Design review of the part built by this model. Coordinates are the model's own, in mm. A direction names the side the tool comes from. Give positions to 0.01 mm unless a question says otherwise; leave off trailing zeros. Write each loop counter-clockwise with the first axis right and the second up, starting at its lowest first coordinate (ties: lowest second). Pieces come first, ordered by that corner, then holes. Notation, with made-up numbers: M 83.5,-8 L 123.5,-8 A27 ccw 123.5,20 Z; hole C 24,58.25 d4. An arc over 180 degrees is marked long. Use one line per item in the form item = value. Start each with the question number.
from build123d import *

# Parameters (mm, degrees)
SKETCH2_W               = 30
SKETCH2_H               = 30
BOSS_EXTRUDE1_DEPTH     = 36
BOSS_EXTRUDE2_DEPTH     = 80
SKETCH5_R               = 4.1
CUT_EXTRUDE1_DEPTH      = 80
CUT_EXTRUDE2_DEPTH      = 80
CUT_EXTRUDE2_DEPTH_BACK = 80
CHAMFER1_SIZE           = 5


with BuildPart() as part:
    # Sketch2 → Boss-Extrude1 (new body)
    with BuildSketch(Plane(origin=(0, 0, 0), x_dir=(1, 0, 0), z_dir=(0, 1, 0))):
        Rectangle(SKETCH2_W, SKETCH2_H)
    extrude(amount=BOSS_EXTRUDE1_DEPTH)

    # Sketch4 → Boss-Extrude2 (add)
    with BuildSketch(Plane(origin=(15, 0, 0), x_dir=(0, 0, -1), z_dir=(1, 0, 0))):
        Polygon((-8.392439038, 4), (-3, 0), (0, 0), (3, 0), (7.607560962, 4), align=None)
    extrude(amount=BOSS_EXTRUDE2_DEPTH)

    # Sketch5 → Cut-Extrude1 (cut)
    with BuildSketch(Plane(origin=(15, 0, 0), x_dir=(0, 0, -1), z_dir=(1, 0, 0))):
        with Locations((0, 9)):
            Circle(SKETCH5_R)
    extrude(amount=-CUT_EXTRUDE1_DEPTH, mode=Mode.SUBTRACT)

    # Sketch6 → Cut-Extrude2 (cut, two sides)
    with BuildSketch(Plane(origin=(15, 0, 0), x_dir=(0, 0, -1), z_dir=(1, 0, 0))) as cut_extrude2_sk:
        with BuildLine():
            Line((2.528554435, 36.330541101), (-2.528554435, 36.330541101))
            Line((-2.528554435, 36.330541101), (-2.528554435, 29.330704688))
            ThreePointArc((-2.528554435, 29.330704688), (-5.755916854, 22.704075168), (0, 18.1))
            ThreePointArc((0, 18.1), (5.755916854, 22.704075168), (2.528554435, 29.330704688))
            Line((2.528554435, 29.330704688), (2.528554435, 36.330541101))
        make_face()
    extrude(amount=CUT_EXTRUDE2_DEPTH, mode=Mode.SUBTRACT)
    extrude(cut_extrude2_sk.sketch, amount=-CUT_EXTRUDE2_DEPTH_BACK, mode=Mode.SUBTRACT)

    # Chamfer1
    chamfer1_edges = [part.edges().sort_by_distance(p)[0] for p in [
        (0, 36, 15),
        (15, 36, -8.764277217),
        (15, 36, 8.764277217),
        (15, 18, 15),
        (15, 18, -15),
        (0, 36, -15),
    ]]
    chamfer(chamfer1_edges, length=CHAMFER1_SIZE)


solid = part.part
1. We need section A-A (y = 9). State the section outline as (x, z) points, and give its area (3 significant figures).
2. For faces 4 (the flat face through (0, 33, 2.529)), 5 (the flat face through (-3, 36, -6)), 6 (the flat face through (54, 4, 0)), list the 3-axis set-ups (+Z, -Z, +X, -X, +Y, -Y) from which the entire face can be reached by the end or side of a thin tool; tool diameter is ignored.
3. Clearance check with flat-ended pins moving along their axes: pin 1 Ø6 at (y, z) = (9, 4) entering from +X; pin 2 Ø10 at (x, z) = (81, 6) entering from +Y; pin 3 Ø12 at (x, z) = (27.5, -0.5) entering from -Y; pin 4 Ø4 at (x, z) = (73.5, -10.5) entering from +Y. State where each tip first meets the part, or that it passes through.
4. Draft analysis for pull direction Z (two halves, no side actions). For faces 1 (the flat face through (54.44, 1.97, -5.27)), 2 (the cylindrical face through (0.2, 5, 0.9)), 3 (the flat face through (11.9, 32.6, 11.5)), state which applies: pulls with the +Z half, pulls with the -Z half, needs draft (parallel to the pull), parting line crosses it, or undercut.
5. To check wall thickness, follow L1, parallel to Z at x = 2, y = 23.5; L2, parallel to X at y = 19.5, z = 7.25; L3, parallel to Z at x = -4, y = 25. State the ranges of each line that lie inside material, in increasing order.
6. We need section C-C (z = 1). State the section outline as (x, y) points.
7. We need section D-D (z = -12). State the section outline as (x, y) points, and give its area (4 significant figures).
8. We need section B-B (x = 12.5). State the section outline as (y, z) points, and give its area (3 significant figures).
Answer block:
q1.outline = M -15,-15 L 10,-15 L 15,-10 L 15,-4.1 L -15,-4.1 Z; M -15,4.1 L 15,4.1 L 15,10 L 10,15 L -15,15 Z
q1.area = 629 mm^2
q2.face_4 = +X, -X, +Y
q2.face_5 = +Z, -Z, +X, -X, +Y
q2.face_6 = +Z, -Z, +X, +Y
q3.pin_1 = 15
q3.pin_2 = 4
q3.pin_3 = 0
q3.pin_4 = through
q4.face_1 = pulls with the -Z half
q4.face_2 = undercut
q4.face_3 = pulls with the +Z half
q5.L1 = -15 to -5.88, 5.88 to 15
q5.L2 = -15 to 15
q5.L3 = -15 to -5.81, 5.81 to 15
q6.outline = M -15,0 L 95,0 L 95,4 L 15,4 L 15,5.02 L -15,5.02 Z; M -15,12.98 L 15,12.98 L 15,18.19 L -15,18.19 Z
q7.outline = M -15,0 L 13,0 L 13,31 L 10,34 L -15,34 Z
q7.area = 947.5 mm^2
q8.outline = M 0,-12.5 L 31,-12.5 L 33.5,-10 L 33.5,-2.53 L 29.33,-2.53 A5.9 cw long 29.33,2.53 L 33.5,2.53 L 33.5,10 L 31,12.5 L 0,12.5 Z; hole C 9,0 d8.2
q8.area = 650 mm^2
